The listing builds one solid part. Answer for the finished solid, in the listing's coordinates (mm). Face numbers are marked on the shaded views. A direction names the side the tool comes from. Give positions to 0.01 mm unless a question says otherwise; leave off trailing zeros. Write each loop counter-clockwise with the first axis right and the second up, starting at its lowest first coordinate (ties: lowest second). Pieces come first, ordered by that corner, then holes. Notation, with made-up numbers: M 10.25,4 L 66.25,4 A19 cw 66.25,18 Z; hole C 14,32.5 d3. An arc over 180 degrees is marked long. Answer as a JSON object with one key per item and string values.
```python
from build123d import *

# Parameters (mm, degrees)
F0_W     = 255.5162906647
F0_H     = 55.8418184519
F1_DEPTH = 25.4
F2_R     = 5.08
F3_R     = 115.1905151489
F4_DEPTH = 25.4


with BuildPart() as f1:
    # F0 (on Top) → F1 (new body)
    with BuildSketch(Plane.XY):
        with Locations((4.1319578886, 4.2407922447)):
            Rectangle(F0_W, F0_H)
    extrude(amount=F1_DEPTH)

    # F2
    f2_edges = [f1.edges().sort_by_distance(p)[0] for p in [
        (-123.626187, 4.240792, 25.4),
        (4.131958, -23.680117, 25.4),
        (131.890103, 4.240792, 25.4),
        (4.131958, 32.161701, 25.4),
    ]]
    fillet(f2_edges, radius=F2_R)

    # F3 (on Front) → F4 (join)
    with BuildSketch(Plane.XZ):
        Circle(F3_R)
    extrude(amount=F4_DEPTH)


solid = f1.part
```
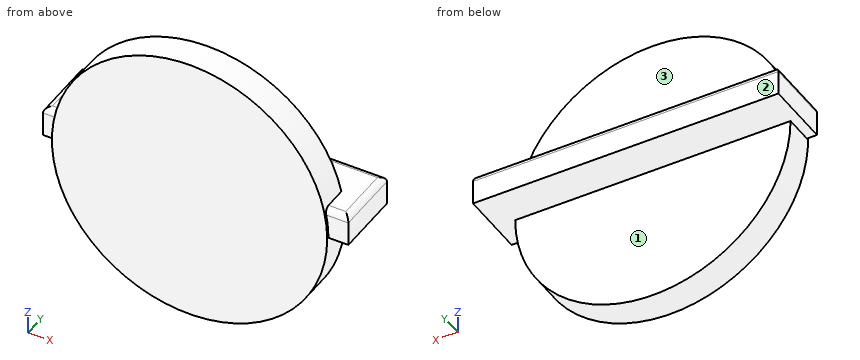
1. A cutting plane is placed at B-B, the plane x = 0.5. Give the vertices of the cut face in (y, z), plus the area to 3 significant figures.
Verdict:
{"outline": "M -25.4,-115.19 L 0,-115.19 L 0,0 L 32.16,0 L 32.16,20.32 A5.08 ccw 27.08,25.4 L 0,25.4 L 0,115.19 L -25.4,115.19 Z", "area": "6,660 mm2"}
2. For the marked faces 1, 2 and 3, determine the directions among +Z, -Z, +X, -X, +Y, -Y from which every point of the face is accessible in a straight line to the end or side of a thin tool.
Verdict:
{"face 1": "-Z, +X, -X, +Y", "face 2": "+Z, -Z, +X, -X, +Y", "face 3": "+Z, +X, -X, +Y"}
3. A cutting plane is placed at C-C, the plane z = 91.5. Give the vertices of the cut face in (x, y).
Verdict:
{"outline": "M -69.98,-25.4 L 69.98,-25.4 L 69.98,0 L -69.98,0 Z"}
4. Consider line 1 along Z through (x, y) = (-54.5, 5.5); line 2 along Y through (x, z) = (75, -50); line 3 along Z through (x, y) = (37.5, -6). Determine where each line is inside the solid, lowest interval first.
Verdict:
{"line 1": "z = 0 to 25.4", "line 2": "y = -25.4 to 0", "line 3": "z = -108.92 to 108.92"}
5. A cutting plane is placed at A-A, the plane y = -5. Give the vertices of the cut face in (x, z), plus the area to 3 significant figures.
Verdict:
{"outline": "M -123.63,0 L -115.19,0 A115.19 ccw 115.19,0 L 131.89,0 L 131.89,20.32 A5.08 ccw 126.81,25.4 L 112.36,25.4 A115.19 ccw -112.36,25.4 L -118.55,25.4 A5.08 ccw -123.63,20.32 Z", "area": "42,400 mm2"}
6. A cutting plane is placed at D-D, the plane x = -98. Give the vertices of the cut face in (y, z).
Verdict:
{"outline": "M -25.4,-60.54 L 0,-60.54 L 0,0 L 32.16,0 L 32.16,20.32 A5.08 ccw 27.08,25.4 L 0,25.4 L 0,60.54 L -25.4,60.54 Z"}
7. Flat-ended cylindrical pins translate along their axes: pin 1 (9.5 mm diameter, centred on x = 120.5, z = 7, fed in from -Y); pin 2 (5 mm diameter, centred on x = 32.5, y = -8.5, fed in from +Z); pin 3 (5 mm diameter, centred on x = 57, y = 16.5, fed in from +Z). Find the tip coordinate at first contact, or state that the pin passes through.
Verdict:
{"pin 1": "stops at y = -23.68", "pin 2": "stops at z = 111.22", "pin 3": "stops at z = 25.4"}
